Design review of the part shown in the three views and the two pictorial views. Dimensions are in mm from the part's minimum x, y and z. Coordinates: 2 decimals unless noted, no trailing zeros. Write each loop counter-clockwise with the first axis right and the second up, starting at its lowest first coordinate (ties: lowest second). Pieces come first, ordered by that corner, then holes. Notation, with made-up numbers: (-3.75, -9.75) - (9.25, -9.75) arc R22 ccw to (9.25, 12.25) - close; hole circle Ø6 at (23.5, 8). An arc over 180 degrees is marked (long way). Return JSON: item names as keys, results as strings. Group by question number.
(1) For pin 1 Ø1.5 at (x, y) = (0.5, 48) entering from -Z, flat-tipped, find the tip position at first contact; note if it passes through.
(2) To check wall thickness, follow L1, parallel to Y at x = 2.95, z = 88.5; L2, parallel to Z at x = 2.6, y = 29.5; L3, parallel to Y at x = 1.55, z = 72.5. State the ranges of each line that lie inside material, in increasing order. Write a range as from..to.
(3) We need section C-C on y = 52. State the section outline as (x, z) points (1 decimal).
(4) We need section B-B on z = 104. State the section outline as (x, y) points (3 decimals).
(5) We need section A-A on x = 1.55. State the section outline as (y, z) points.
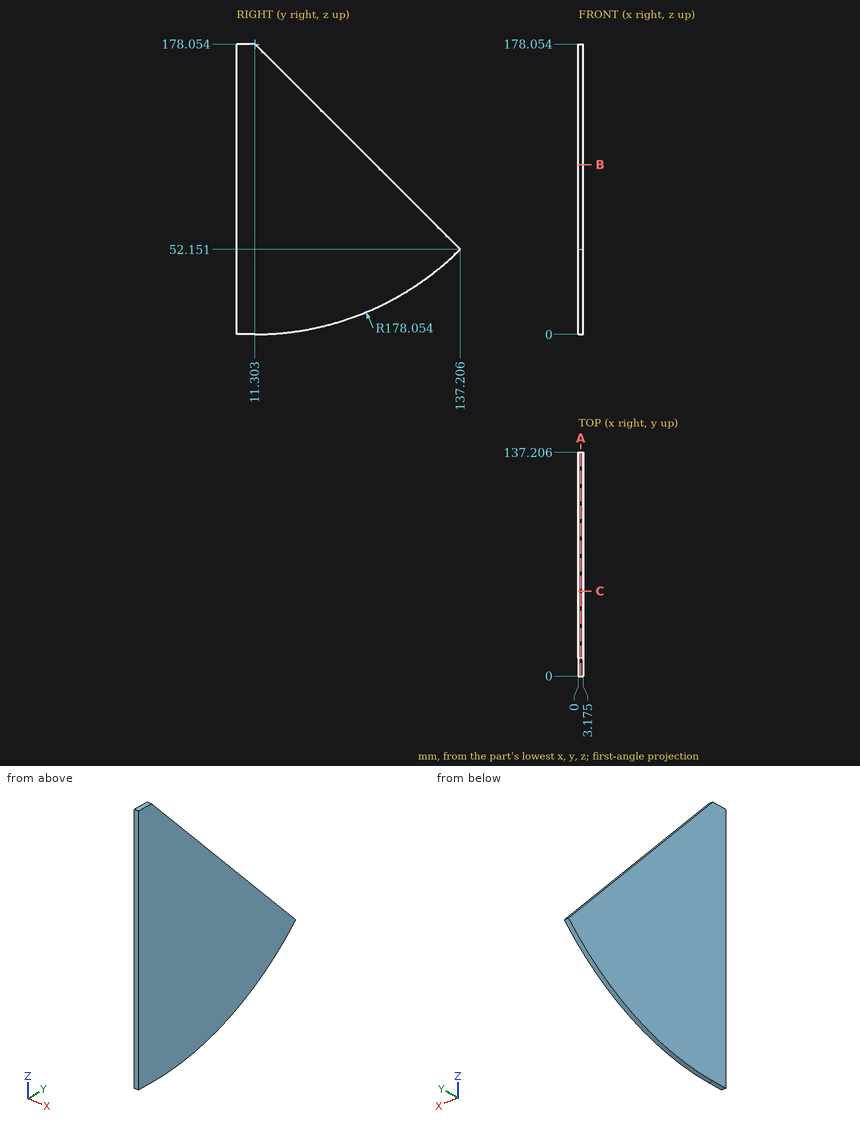
Ans:
{
 "1": {"pin 1": "z = 3.67"},
 "2": {"L1": "0..100.86", "L2": "0.93..159.86", "L3": "0..116.86"},
 "3": {"outline": "(0, 4.7) - (3.2, 4.7) - (3.2, 137.4) - (0, 137.4) - close"},
 "4": {"outline": "(0, 0) - (3.175, 0) - (3.175, 85.357) - (0, 85.357) - close"},
 "5": {"outline": "(0, 0) - (11.3, 0) arc R178.05 ccw to (137.21, 52.15) - (11.3, 178.05) - (0, 178.05) - close"}
}
